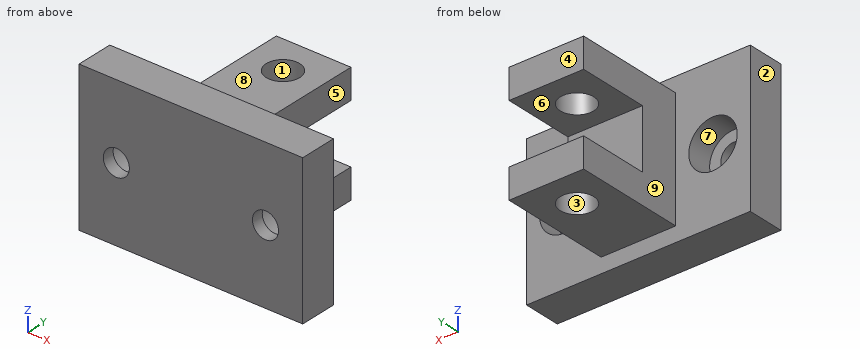
```python
from build123d import *

# Parameters (mm, degrees)
SKETCH1_W                                           = 30
SKETCH1_H                                           = 20
BOSS_EXTRUDE1_DEPTH                                 = 5
SKETCH2_W                                           = 10
SKETCH2_H                                           = 16
BOSS_EXTRUDE2_DEPTH                                 = 15
SKETCH3_W                                           = 8
SKETCH3_H                                           = 9.586057572
CUT_EXTRUDE1_DEPTH                                  = 31
SKETCH4_R                                           = 2.25
CUT_EXTRUDE2_DEPTH                                  = 31.805843601
SKETCH5_R                                           = 1.75
CUT_EXTRUDE3_DEPTH                                  = 15
CBORE_FOR_M3_HEX_SOCKET_HEAD_CAP_SCREW1_D           = 3.4
CBORE_FOR_M3_HEX_SOCKET_HEAD_CAP_SCREW1_CBORE_D     = 6.5
CBORE_FOR_M3_HEX_SOCKET_HEAD_CAP_SCREW1_CBORE_DEPTH = 3.4


with BuildPart() as part:
    # Sketch1 → Boss-Extrude1 (new body)
    with BuildSketch(Plane(origin=(0, 0, 0), x_dir=(1, 0, 0), z_dir=(0, 1, 0))):
        Rectangle(SKETCH1_W, SKETCH1_H)
    extrude(amount=BOSS_EXTRUDE1_DEPTH)

    # Sketch2 → Boss-Extrude2 (add)
    with BuildSketch(Plane(origin=(0, 5, 0), x_dir=(1, 0, 0), z_dir=(0, 1, 0))):
        Rectangle(SKETCH2_W, SKETCH2_H)
    extrude(amount=BOSS_EXTRUDE2_DEPTH)

    # Sketch3 → Cut-Extrude1 (cut, through all)
    with BuildSketch(Plane.ZY.offset(5)):
        with Locations((0, 15.206971214)):
            Rectangle(SKETCH3_W, SKETCH3_H)
    extrude(amount=-CUT_EXTRUDE1_DEPTH, mode=Mode.SUBTRACT)

    # Sketch4 → Cut-Extrude2 (cut, through all)
    with BuildSketch(Plane(origin=(0, 0, -8), x_dir=(-1, 0, 0), z_dir=(0, 0, -1))):
        with Locations((0, 15)):
            Circle(SKETCH4_R)
    extrude(amount=-CUT_EXTRUDE2_DEPTH, mode=Mode.SUBTRACT)

    # Sketch5 → Cut-Extrude3 (cut)
    with BuildSketch(Plane(origin=(0, 5, 0), x_dir=(1, 0, 0), z_dir=(0, 1, 0))):
        with Locations(Location((-10, 0, 0), (0, 0, 270))):
            Circle(SKETCH5_R)
        with Locations(Location((10, 0, 0), (0, 0, 270))):
            Circle(SKETCH5_R)
    extrude(amount=-CUT_EXTRUDE3_DEPTH, mode=Mode.SUBTRACT)

    # CBORE for M3 Hex Socket Head Cap Screw1 (through all)
    with Locations(Plane(origin=(0, 5, 0), x_dir=(1, 0, 0), z_dir=(0, 1, 0))):
        with Locations((-10, 0), (10, 0)):
            CounterBoreHole(CBORE_FOR_M3_HEX_SOCKET_HEAD_CAP_SCREW1_D / 2, CBORE_FOR_M3_HEX_SOCKET_HEAD_CAP_SCREW1_CBORE_D / 2, CBORE_FOR_M3_HEX_SOCKET_HEAD_CAP_SCREW1_CBORE_DEPTH)


solid = part.part
```
The model under review builds one solid part; all positions refer to its coordinate system, in mm. Face numbers are marked on the shaded views. A direction names the side the tool comes from. Round coordinates to 2 decimals unless told otherwise and drop trailing zeros. Write each loop counter-clockwise with the first axis right and the second up, starting at its lowest first coordinate (ties: lowest second). Pieces come first, ordered by that corner, then holes. Notation, with made-up numbers: M 45,-29 L 60,-29 A19 cw 60,-17 Z; hole C 46.5,11.5 d1. An arc over 180 degrees is marked long. Use CSV: the item, a comma, the result in double quotes. Start each with the question number.
(1) Tool access review of the marked faces 5, 6, 7, 8 and 9: name each direction out of +Z, -Z, +X, -X, +Y, -Y from which nothing blocks a thin tool from reaching the whole face with its end or side.
(2) Clearance check with flat-ended pins moving along their axes: P1, Ø7.5, axis at x = 10, z = 0, coming from the +Y side; P2, Ø8, axis at x = -2.5, y = 15, coming from the -Z side; P3, Ø6, axis at y = 11.5, z = 2.5, coming from the -X side; P4, Ø1.5, axis at x = -8.5, z = -7, coming from the -Y side. State where each tip first meets the part, or that it passes through.
(3) We need section C-C, the plane y = 15. State the section outline as (x, z) points.
(4) We need section D-D, the plane x = 0. State the section outline as (y, z) points, then the cut area to 3 significant figures.
(5) For line 1 along X through (y, z) = (0.5, 0); line 2 along Y through (x, z) = (0, -5.45); line 3 along Z through (x, y) = (-10, 2.8), list the stretches that pass through material, from the lowest coordinate up.
(6) The part is to be moulded in two halves that separate along X. For the marked faces 1, 2, 3 and 4, say which applies: +X half, -X half, draft (parallel to the pull), parting line (faces both ways), or undercut.
(7) We need section A-A, the plane x = 10. State the section outline as (y, z) points, then the cut area to 3 significant figures.
(8) We need section B-B, the plane z = 0. State the section outline as (x, y) points.
Findings:
1,face 5,"+Z, -Z, +X, +Y"
1,face 6,"+X, -X, +Y"
1,face 7,"+Y"
1,face 8,"+Z, +X, -X, +Y"
1,face 9,"+Z, -Z, -X, +Y"
2,P1,"y = 5"
2,P2,"z = -8"
2,P3,"x = -5"
2,P4,"y = 0"
3,outline,"M -5,-8 L -2.25,-8 L -2.25,-4 L -5,-4 Z; M -5,4 L -2.25,4 L -2.25,8 L -5,8 Z; M 2.25,-8 L 5,-8 L 5,-4 L 2.25,-4 Z; M 2.25,4 L 5,4 L 5,8 L 2.25,8 Z"
4,outline,"M 0,-10 L 5,-10 L 5,-8 L 12.75,-8 L 12.75,-4 L 10.41,-4 L 10.41,4 L 12.75,4 L 12.75,8 L 5,8 L 5,10 L 0,10 Z; M 17.25,-8 L 20,-8 L 20,-4 L 17.25,-4 Z; M 17.25,4 L 20,4 L 20,8 L 17.25,8 Z"
4,area,"227 mm^2"
5,line 1,"-15 to -11.75, -8.25 to 8.25, 11.75 to 15"
5,line 2,"0 to 12.75, 17.25 to 20"
5,line 3,"-10 to -3.25, 3.25 to 10"
6,face 1,"undercut"
6,face 2,"-X half"
6,face 3,"undercut"
6,face 4,"draft"
7,outline,"M 0,-10 L 5,-10 L 5,-3.25 L 1.6,-3.25 L 1.6,-1.75 L 0,-1.75 Z; M 0,1.75 L 1.6,1.75 L 1.6,3.25 L 5,3.25 L 5,10 L 0,10 Z"
7,area,"72.3 mm^2"
8,outline,"M -15,0 L -11.75,0 L -11.75,1.6 L -13.25,1.6 L -13.25,5 L -15,5 Z; M -8.25,0 L 8.25,0 L 8.25,1.6 L 6.75,1.6 L 6.75,5 L 5,5 L 5,10.41 L -5,10.41 L -5,5 L -6.75,5 L -6.75,1.6 L -8.25,1.6 Z; M 11.75,0 L 15,0 L 15,5 L 13.25,5 L 13.25,1.6 L 11.75,1.6 Z"
